Source: CAD feature listing. Evaluate the final solid. Frame: model axes, mm. A direction names the side the tool comes from. Give positions to 0.01 mm unless a question says otherwise; leave off trailing zeros. Loops run counter-clockwise (first coordinate to the right, second up) from the corner with the lowest first, then second, coordinate; pieces in that order, holes last. Notation, with made-up numbers: (69.5, 44) -> (112.5, 44) arc R21 cw to (112.5, 60) -> close; hole circle Ø4 at (12.5, 74). An arc over 180 degrees is marked (long way). Return JSON: item names as keys, results as strings. Group by question number.
(1) Draft query along X for faces 4 (the face through (36.57, -36.5, 0.37)), 5 (the face through (37, 0, 0)), 6 (the face through (-32.57, -32.5, 0.37)). Return one class per face: released by +X, released by -X, zero draft, split by the parting line, or undercut.
(2) Ray query, line 1 (Y direction, x = 26.5, z = 0.25); line 2 (X direction, y = 16, z = 0.9); line 3 (X direction, y = 17, z = 1.4). Return the intervals inside material, ascending. Write a range as from..to.
(3) Cut plane C-C on z = 1.45. Return loops of the section in (x, y).
(4) Access query for faces 1 (the face through (-0.462, -37.501, 1.974)), 2 (the face through (-32.5, 32.57, 0.37)), 3 (the face through (-0.406, 34.499, 1.974)). Directions: +Z, -Z, +X, -X, +Y, -Y. A direction counts if a zero-diameter tool reaches every point of the face in a straight line with its end or side. Return the directions, or none.
(5) Cut plane A-A on y = -1.5. Return loops of the section in (x, z), then the cut area to 3 significant figures.
```python
from build123d import *

# Parameters (mm, degrees)
BOSS_EXTRUDE1_DEPTH = 2.5
FILLET1_R           = 1.75


with BuildPart() as part:
    # Sketch1 → Boss-Extrude1 (new body)
    with BuildSketch(Plane.XY):
        with BuildLine():
            Line((-33, 38), (33, 38))
            ThreePointArc((33, 38), (36.535533906, 36.535533906), (38, 33))
            Line((38, 33), (38, -33))
            ThreePointArc((38, -33), (36.535533906, -36.535533906), (33, -38))
            Line((33, -38), (-33, -38))
            ThreePointArc((-33, -38), (-36.535533906, -36.535533906), (-38, -33))
            Line((-38, -33), (-38, 33))
            ThreePointArc((-38, 33), (-36.535533906, 36.535533906), (-33, 38))
        make_face()
        with BuildLine():
            Line((29, 34), (-29, 34))
            ThreePointArc((-29, 34), (-32.535533906, 32.535533906), (-34, 29))
            Line((-34, 29), (-34, -29))
            ThreePointArc((-34, -29), (-32.535533906, -32.535533906), (-29, -34))
            Line((-29, -34), (29, -34))
            ThreePointArc((29, -34), (32.535533906, -32.535533906), (34, -29))
            Line((34, -29), (34, 29))
            ThreePointArc((34, 29), (32.535533906, 32.535533906), (29, 34))
        make_face(mode=Mode.SUBTRACT)
    extrude(amount=BOSS_EXTRUDE1_DEPTH)

    # Fillet1
    fillet1_edges = [part.edges().sort_by_distance(p)[0] for p in [
        (36.535533906, -36.535533906, 2.5),
        (38, 0, 2.5),
        (36.535533906, 36.535533906, 2.5),
        (0, 38, 2.5),
        (-36.535533906, 36.535533906, 2.5),
        (-38, 0, 2.5),
        (-32.535533906, -32.535533906, 2.5),
        (0, -34, 2.5),
        (32.535533906, -32.535533906, 2.5),
        (34, 0, 2.5),
        (32.535533906, 32.535533906, 2.5),
        (0, 34, 2.5),
        (-32.535533906, 32.535533906, 2.5),
        (-34, 0, 2.5),
        (-36.535533906, -36.535533906, 2.5),
        (0, -38, 2.5),
    ]]
    fillet(fillet1_edges, radius=FILLET1_R)


solid = part.part
```
Answers:
{
 "1": {"face 4": "released by +X", "face 5": "zero draft", "face 6": "undercut"},
 "2": {"line 1": "-38..-34, 34..38", "line 2": "-37.99..-34.01, 34.01..37.99", "line 3": "-37.87..-34.13, 34.13..37.87"},
 "3": {"outline": "(-37.85, -33) arc R4.85 ccw to (-33, -37.85) -> (33, -37.85) arc R4.85 ccw to (37.85, -33) -> (37.85, 33) arc R4.85 ccw to (33, 37.85) -> (-33, 37.85) arc R4.85 ccw to (-37.85, 33) -> close; hole (-34.15, -29) arc R5.15 ccw to (-29, -34.15) -> (29, -34.15) arc R5.15 ccw to (34.15, -29) -> (34.15, 29) arc R5.15 ccw to (29, 34.15) -> (-29, 34.15) arc R5.15 ccw to (-34.15, 29) -> close"},
 "4": {"face 1": "+Z, +X, -X, -Y", "face 2": "+Z, -Z", "face 3": "+Z"},
 "5": {"outline": "(-38, 0) -> (-34, 0) -> (-34, 0.75) arc R1.75 ccw to (-35.75, 2.5) -> (-36.25, 2.5) arc R1.75 ccw to (-38, 0.75) -> close; (34, 0) -> (38, 0) -> (38, 0.75) arc R1.75 ccw to (36.25, 2.5) -> (35.75, 2.5) arc R1.75 ccw to (34, 0.75) -> close", "area": "17.4 mm²"}
}
